Geometry: final body of the model. Coordinates: model frame, mm. A direction names the side the tool comes from. Coordinates: 2 decimals unless noted, no trailing zeros. Order: outer loops, then holes, each group sorted by start corner. A loop starts at its lowest first (then second) coordinate and runs counter-clockwise, first axis right, second up. Notation, with made-up numbers: (-33, -3.75) - (23, -3.75) arc R18 ccw to (23, 29.25) - close; hole circle Ø9 at (-13.5, 73). An arc over 180 degrees is marked (long way). Use a Markdown table: item, result. Add a question column.
```python
from build123d import *

# Parameters (mm, degrees)
BOSS_EXTRU_1_DEPTH           = 5
BOSS_EXTRU_1_DEPTH_BACK      = 5
TROU_TARAUD_M81_D            = 6.8
ESQUISSE5_R                  = 1.5
ENL_V_MAT_EXTRU_1_DEPTH      = 60.476400504
R_P_TITION_CIRCULAIRE1_COUNT = 3


with BuildPart() as part:
    # Esquisse1 → Boss.-Extru.1 (new, two sides: drawn at the far end of the back side and taken through both)
    with BuildSketch(Plane(origin=(0, 0, 0), x_dir=(0, 0, -1), z_dir=(1, 0, 0)).offset(-BOSS_EXTRU_1_DEPTH_BACK)):
        with BuildLine():
            Line((-3, 42.5), (3, 42.5))
            Line((3, 42.5), (3, 19.773719933))
            ThreePointArc((3, 19.773719933), (17.320508076, 10), (18.62454379, -7.288783755))
            Line((18.62454379, -7.288783755), (38.306079661, -18.651923789))
            Line((38.306079661, -18.651923789), (35.306079661, -23.848076211))
            Line((35.306079661, -23.848076211), (15.62454379, -12.484936178))
            ThreePointArc((15.62454379, -12.484936178), (0, -20), (-15.62454379, -12.484936178))
            Line((-15.62454379, -12.484936178), (-35.306079661, -23.848076211))
            Line((-35.306079661, -23.848076211), (-38.306079661, -18.651923789))
            Line((-38.306079661, -18.651923789), (-18.62454379, -7.288783755))
            ThreePointArc((-18.62454379, -7.288783755), (-17.320508076, 10), (-3, 19.773719933))
            Line((-3, 19.773719933), (-3, 42.5))
        make_face()
    extrude(amount=BOSS_EXTRU_1_DEPTH + BOSS_EXTRU_1_DEPTH_BACK)

    # Trou taraudé M81 (through all)
    with Locations(Plane(origin=(5, 0, 0), x_dir=(0, 0, -1), z_dir=(1, 0, 0))):
        with Locations((0, 0)):
            Hole(TROU_TARAUD_M81_D / 2)

    # Esquisse5 → Enlèv. mat.-Extru.1 (cut, through all)
    with BuildSketch(Plane.XY.offset(3)):
        with Locations((0, 37.5)):
            Circle(ESQUISSE5_R)
        with BuildLine():
            Line((-5, 19.773719933), (-5, 37.5))
            ThreePointArc((-5, 37.5), (0, 42.5), (5, 37.5))
            Line((5, 37.5), (5, 19.773719933))
            Line((5, 19.773719933), (13.62028311, 19.773719933))
            Line((13.62028311, 19.773719933), (13.62028311, 47.5))
            Line((13.62028311, 47.5), (-13.199246966, 47.5))
            Line((-13.199246966, 47.5), (-13.199246966, 19.773719933))
            Line((-13.199246966, 19.773719933), (-5, 19.773719933))
        make_face()
    enl_v_mat_extru_1 = extrude(amount=-ENL_V_MAT_EXTRU_1_DEPTH, mode=Mode.SUBTRACT)

    # Répétition circulaire1: Enlèv. mat.-Extru.1 ×3 about axis
    r_p_tition_circulaire1_axis = Axis((5, 0, 0), (1, 0, 0))
    for i in range(1, R_P_TITION_CIRCULAIRE1_COUNT):
        add(enl_v_mat_extru_1.rotate(r_p_tition_circulaire1_axis, i * 360 / R_P_TITION_CIRCULAIRE1_COUNT), mode=Mode.SUBTRACT)


solid = part.part
```
1) First-contact query: pin 1 (4 mm diameter, centred on x = -1, y = -7, fed in from -Z); pin 2 (5 mm diameter, centred on x = 2, y = 34.5, fed in from +Z); pin 3 (3.5 mm diameter, centred on x = 0, y = 37.5, fed in from -Z). Flat tips, straight axial feed; report the tip coordinate or a pass-through.
2) Line query: line 1 (Y direction, x = 0, z = -0.4); line 2 (Y direction, x = 0, z = 0.8); line 3 (Z direction, x = 3.75, y = -16). Output: solid intervals per line, ascending. Write a range as from..to.
3) Draft query along Z for faces 4 (the cylindrical face through (0, 36, 0)), 5 (the flat face through (-0.07, -18.246, -25.603)), 6 (the flat face through (0, 31, 3)). Return one class per face: released by +Z, released by -Z, zero draft, split by the parting line, or undercut.
4) Section query B-B (x = -0.25). Return the cut outline in (y, z), and give its area (3 significant figures).
5) Access query for faces 1 (the flat face through (-0.07, -18.09, 25.33)), 2 (the flat face through (5, -5, 0)), 3 (the flat face through (0, 31, -3)). Directions: +Z, -Z, +X, -X, +Y, -Y. A direction counts if a zero-diameter tool reaches every point of the face in a straight line with its end or side. Return the directions, or none.
6) Section query C-C (x = 3.5). Return the cut outline in (y, z).
7) Section query D-D (y = 27.5). Return the cut outline in (x, z).
8) Section query A-A (z = 0). Return the cut outline in (x, y).
From the geometry:
| question | item | result |
|---|---|---|
| 1 | pin 1 | stops at z = -21.59 |
| 1 | pin 2 | stops at z = 3 |
| 1 | pin 3 | stops at z = -3 |
| 2 | line 1 | y = -20..-3.38, 3.38..36, 39..42.5 |
| 2 | line 2 | y = -19.98..-3.3, 3.3..36, 39..42.5 |
| 2 | line 3 | z = -33.71..-21.71, -12..12, 21.71..33.71 |
| 3 | face 4 | zero draft |
| 3 | face 5 | undercut |
| 3 | face 6 | released by +Z |
| 4 | outline | (-23.84, -35.3) - (-18.65, -38.3) - (-16.89, -35.26) - (-22.09, -32.26) - close; (-23.84, 35.3) - (-22.09, 32.26) - (-16.89, 35.26) - (-18.65, 38.3) - close; (-20.61, -29.7) - (-15.41, -32.7) - (-7.29, -18.62) arc R20 ccw to (19.77, -3) - (36.02, -3) - (36.02, 3) - (19.77, 3) arc R20 ccw to (-7.29, 18.62) - (-15.41, 32.7) - (-20.61, 29.7) - (-12.48, 15.62) arc R20 ccw to (-12.48, -15.62) - close; (38.98, -3) - (42.49, -3) - (42.49, 3) - (38.98, 3) - close; hole circle Ø6.8 at (0, 0) |
| 4 | area | 1,570 mm^2 |
| 5 | face 1 | +X, -X, -Y |
| 5 | face 2 | +Z, -Z, +X, +Y, -Y |
| 5 | face 3 | -Z, +X, -X, +Y |
| 6 | outline | (-23.13, -34.07) - (-17.94, -37.07) - (-7.29, -18.62) arc R20 ccw to (19.77, -3) - (41.07, -3) - (41.07, 3) - (19.77, 3) arc R20 ccw to (-7.29, 18.62) - (-17.94, 37.07) - (-23.13, 34.07) - (-12.48, 15.62) arc R20 ccw to (-12.48, -15.62) - close; hole circle Ø6.8 at (0, 0) |
| 7 | outline | (-5, -3) - (5, -3) - (5, 3) - (-5, 3) - close |
| 8 | outline | (-5, -20) - (5, -20) - (5, -3.4) - (-5, -3.4) - close; (-5, 3.4) - (5, 3.4) - (5, 37.5) arc R5 ccw to (-5, 37.5) - close; hole circle Ø3 at (0, 37.5) |
